from build123d import *

# Parameters (mm, degrees)
SKETCH1_W                = 50
SKETCH1_H                = 60
BOSS_EXTRUDE1_DEPTH      = 25
CUT_EXTRUDE1_START       = -10
SKETCH2_R                = 22.5
CUT_EXTRUDE1_DEPTH       = 30
SKETCH3_R                = 7.5
CUT_EXTRUDE2_DEPTH       = 64.442887702
SKETCH4_R                = 10
CUT_EXTRUDE3_DEPTH       = 10
SKETCH5_R                = 1.75
CUT_EXTRUDE4_DEPTH       = 10
CHAMFER1_SIZE            = 5
SKETCH6_R                = 2
CUT_EXTRUDE5_DEPTH       = 10
SKETCH7_W                = 11
SKETCH7_H                = 5.906734889
CUT_EXTRUDE6_DEPTH       = 9
CHAMFER2_SIZE            = 5
CHAMFER2_OF_MIRROR1_SIZE = 5
CHAMFER3_SIZE            = 3
CUT_EXTRUDE8_START       = 25
SKETCH10_R               = 2
CUT_EXTRUDE8_DEPTH       = 25.371044267
SKETCH11_R               = 2
CUT_EXTRUDE9_DEPTH       = 50.371044267


with BuildPart() as part:
    # Sketch1 → Boss-Extrude1 (new body)
    with BuildSketch(Plane(origin=(0, 0, 0), x_dir=(1, 0, 0), z_dir=(0, 1, 0))):
        Rectangle(SKETCH1_W, SKETCH1_H)
    extrude(amount=BOSS_EXTRUDE1_DEPTH)

    # Sketch2 → Cut-Extrude1 (cut)
    with BuildSketch(Plane.ZY.offset(25).offset(CUT_EXTRUDE1_START)):
        with Locations((0, 25)):
            Circle(SKETCH2_R)
    extrude(amount=-CUT_EXTRUDE1_DEPTH, mode=Mode.SUBTRACT)

    # Sketch3 → Cut-Extrude2 (cut, through all)
    with BuildSketch(Plane.ZY.offset(25)):
        with Locations((0, 25)):
            Circle(SKETCH3_R)
    extrude(amount=-CUT_EXTRUDE2_DEPTH, mode=Mode.SUBTRACT)

    # Sketch4 → Cut-Extrude3 (cut)
    with BuildSketch(Plane.XY.offset(30)):
        with Locations((0, 25)):
            Circle(SKETCH4_R)
    extrude(amount=-CUT_EXTRUDE3_DEPTH, mode=Mode.SUBTRACT)

    # Sketch5 → Cut-Extrude4 (cut)
    with BuildSketch(Plane.XZ):
        with Locations(Location((-10, 20, 0), (0, 0, 270))):
            Circle(SKETCH5_R)
        with Locations(Location((10, 20, 0), (0, 0, 270))):
            Circle(SKETCH5_R)
        with Locations(Location((-10, -20, 0), (0, 0, 270))):
            Circle(SKETCH5_R)
        with Locations(Location((10, -20, 0), (0, 0, 270))):
            Circle(SKETCH5_R)
    extrude(amount=-CUT_EXTRUDE4_DEPTH, mode=Mode.SUBTRACT)

    # Chamfer1
    chamfer1_edges = [part.edges().sort_by_distance(p)[0] for p in [
        (0, 0, -30),
    ]]
    chamfer(chamfer1_edges, length=CHAMFER1_SIZE)

    # Sketch6 → Cut-Extrude5 (cut)
    with BuildSketch(Plane(origin=(0, 0, -30), x_dir=(-1, 0, 0), z_dir=(0, 0, -1))):
        with Locations((-20, 15)):
            Circle(SKETCH6_R)
        with Locations((20, 15)):
            Circle(SKETCH6_R)
    extrude(amount=-CUT_EXTRUDE5_DEPTH, mode=Mode.SUBTRACT)

    # Sketch7 → Cut-Extrude6 (cut)
    with BuildSketch(Plane(origin=(25, 0, 0), x_dir=(0, 0, -1), z_dir=(1, 0, 0))):
        with Locations((-10, 2.953367444)):
            Rectangle(SKETCH7_W, SKETCH7_H)
        with Locations((10, 2.953367444)):
            Rectangle(SKETCH7_W, SKETCH7_H)
    cut_extrude6 = extrude(amount=-CUT_EXTRUDE6_DEPTH, mode=Mode.SUBTRACT)

    # Chamfer2
    chamfer2_edges = [part.edges().sort_by_distance(p)[0] for p in [
        (16, 5.906734889, 10),
        (16, 5.906734889, -10),
    ]]
    chamfer(chamfer2_edges, length=CHAMFER2_SIZE)

    # Mirror1: Cut-Extrude6 across plane
    add(cut_extrude6.mirror(Plane(origin=(0, 0, 0), x_dir=(0, 0, 1), z_dir=(1, 0, 0))), mode=Mode.SUBTRACT)

    # Chamfer2 of Mirror1
    chamfer2_of_mirror1_edges = [part.edges().sort_by_distance(p)[0] for p in [
        (-16, 5.906734889, 10),
        (-16, 5.906734889, -10),
    ]]
    chamfer(chamfer2_of_mirror1_edges, length=CHAMFER2_OF_MIRROR1_SIZE)

    # Chamfer3
    chamfer3_edges = [part.edges().sort_by_distance(p)[0] for p in [
        (-25, 15, -30),
        (25, 15, -30),
    ]]
    chamfer(chamfer3_edges, length=CHAMFER3_SIZE - 0.0001)  # a hair under: the kernel refuses the full size

    # Sketch10 → Cut-Extrude8 (cut, through all)
    with BuildSketch(Plane(origin=(0, -2.5, -2.5), x_dir=(1, 0, 0), z_dir=(0, 0.7071067811865475, 0.7071067811865477)).offset(CUT_EXTRUDE8_START)):
        with Locations(Location((-20, 1.464466094, 0), (0, 0, 90))):
            Circle(SKETCH10_R)
        with Locations(Location((20, 1.464466094, 0), (0, 0, 90))):
            Circle(SKETCH10_R)
    cut_extrude8 = extrude(amount=CUT_EXTRUDE8_DEPTH, mode=Mode.SUBTRACT)

    # Mirror2: Cut-Extrude8 across plane
    add(cut_extrude8.mirror(Plane.XY), mode=Mode.SUBTRACT)

    # Sketch11 → Cut-Extrude9 (cut, through all)
    with BuildSketch(Plane(origin=(0, -2.5, -2.5), x_dir=(1, 0, 0), z_dir=(0, 0.7071067811865475, 0.7071067811865477))):
        with Locations(Location((17, -14.213203436, 0), (0, 0, 90))):
            Circle(SKETCH11_R)
    extrude(amount=CUT_EXTRUDE9_DEPTH, mode=Mode.SUBTRACT)


solid = part.part
Here's how the part is built. I have some questions about the finished solid (model axes, mm). A direction names the side the tool comes from. Give positions to 0.01 mm unless a question says otherwise; leave off trailing zeros. Loops run counter-clockwise (first coordinate to the right, second up) from the corner with the lowest first, then second, coordinate; pieces in that order, holes last. Notation, with made-up numbers: (-34, 64) -> (17, 64) arc R16 ccw to (17, 81) -> close; hole circle Ø7 at (82.25, 21). An arc over 180 degrees is marked (long way). Answer as a JSON object with one key per item and string values. Group by question number.
Item 1: Imagine slicing it at A-A on y = 20. Give the number of separate pieces and of enclosed holes in the cut face, then the cut area to 3 significant figures.
Item 2: I need wall thicknesses on L1, parallel to X at y = 6.75, z = 20; L2, parallel to X at y = 21, z = -12.5; L3, parallel to X at y = 17.75, z = 13. Which ranges of each line are inside material? Lowest first, please.
Item 3: Imagine slicing it at B-B on z = 0. Write out the boundary of the cut face in (x, y).
Item 4: Will these pins go through, and if not, where does the flat tip stop? pin 1 (0.5 mm diameter, centred on y = 0.5, z = -8, fed in from -X); pin 2 (0.5 mm diameter, centred on y = 0.5, z = 11, fed in from +X); pin 3 (3 mm diameter, centred on x = -23, z = 12, fed in from -Y).
Item 5: Thinking about a two-plate mould opening in Z: for faces 5 (the flat face through (-23, 13, -29)), 6 (the flat face through (0, 12, 30)), 7 (the flat face through (-20.028, 16.193, -14.162)), which applies, pulls with the +Z half, pulls with the -Z half, needs draft (parallel to the pull), parting line crosses it, or undercut?
Item 6: On a 3-axis mill with a long thin cutter (end or side, diameter ignored), from which of +Z, -Z, +X, -X, +Y, -Y can I reach the whole of each face in a straight line? I mean faces 1 (the flat face through (22, 2, -15.5)), 2 (the flat face through (-18.535, 3.442, 10.077)), 3 (the flat face through (19.972, 16.193, -14.162)), 4 (the cylindrical face through (-20, 17, -25)). Say none if no direction works.
Item 7: Imagine slicing it at C-C on x = 20. Write out the boundary of the cut face in (y, z), then the cut area to 3 significant figures.
Answer list:
{
 "1": {"separate pieces": "3", "enclosed holes": "4", "area": "1,240 mm2"},
 "2": {"L1": "x = -25 to -11.75, -8.25 to 8.25, 11.75 to 25", "L2": "x = -25 to -15, 15 to 25", "L3": "x = -25 to -20.64, -19.36 to -15, 15 to 19.36, 20.64 to 25"},
 "3": {"outline": "(-25, 0) -> (25, 0) -> (25, 17.5) -> (15, 17.5) -> (15, 2.5) -> (-15, 2.5) -> (-15, 17.5) -> (-25, 17.5) -> close"},
 "4": {"pin 1": "stops at x = -16", "pin 2": "stops at x = 16", "pin 3": "stops at y = 5.91"},
 "5": {"face 5": "pulls with the -Z half", "face 6": "pulls with the +Z half", "face 7": "undercut"},
 "6": {"face 1": "+X, -Y", "face 2": "-X, -Y", "face 3": "none", "face 4": "-Z"},
 "7": {"outline": "(0, -25) -> (5, -30) -> (13, -30) -> (13, -20) -> (17, -20) -> (17, -30) -> (25, -30) -> (25, -25.76) -> (14.8, -15.56) -> (17.63, -12.73) -> (25, -20.1) -> (25, -7.5) arc R7.5 cw to (25, 7.5) -> (25, 20.1) -> (17.63, 12.73) -> (14.8, 15.56) -> (25, 25.76) -> (25, 30) -> (0, 30) -> (0, 15.5) -> (4.91, 15.5) -> (4.91, 4.5) -> (0, 4.5) -> (0, -4.5) -> (4.91, -4.5) -> (4.91, -15.5) -> (0, -15.5) -> close", "area": "1,150 mm2"}
}
